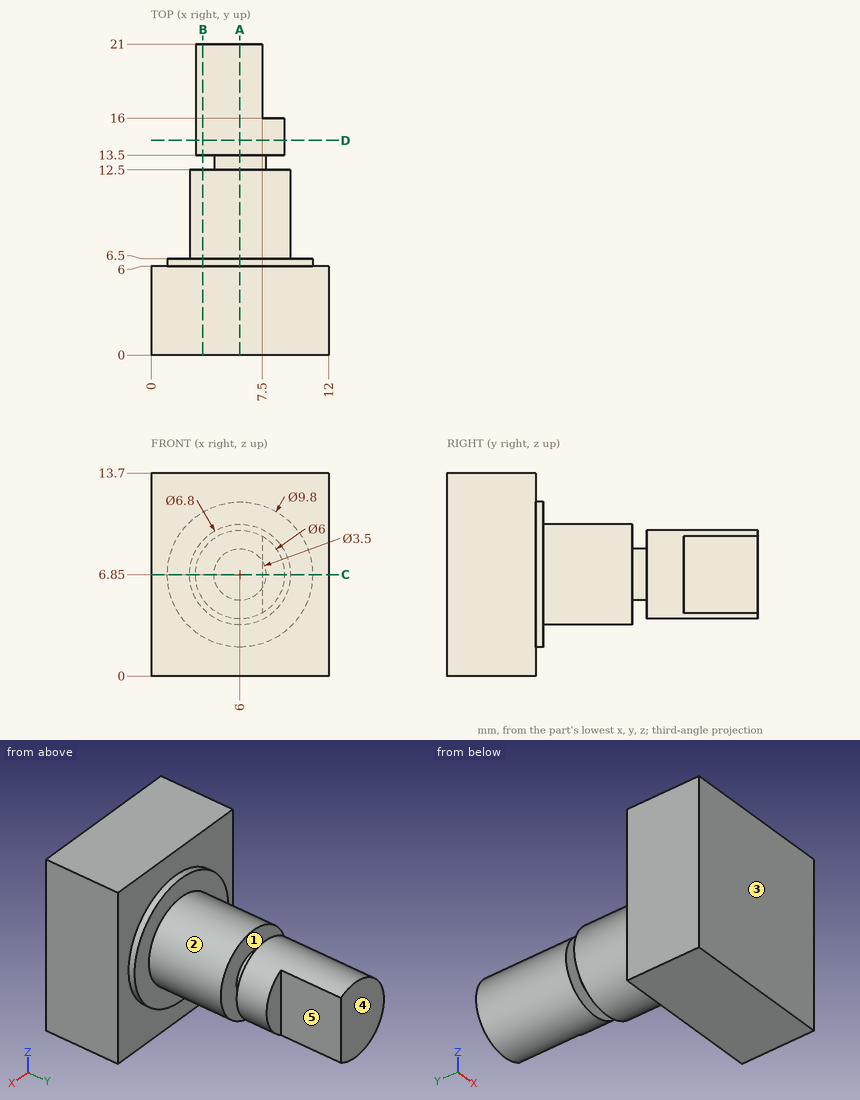
Part print with two shaded views. Sizes in mm from the minimum x, y, z corner. A direction names the side the tool comes from. Give positions to 0.01 mm unless a question says otherwise; leave off trailing zeros. Order: outer loops, then holes, each group sorted by start corner. A loop starts at its lowest first (then second) coordinate and runs counter-clockwise, first axis right, second up.
(1) Tool access for the marked faces 1, 2, 3, 4 and 5: list every direction of +Z, -Z, +X, -X, +Y, -Y with a clear straight run to the whole face (end or side of a thin tool).
(2) Saw through at C-C, the plane z = 6.85. Give the cut face in (x, y), then the cut area to 3 significant figures.
(3) Saw through at D-D, the plane y = 14.5. Give the cut face in (x, z), then the cut area to 3 significant figures.
(4) Drill centre lines: L1, parallel to Y at x = 5.25, z = 1.5; L2, parallel to Y at x = 7.25, z = 4.25; L3, parallel to Y at x = 1.5, z = 5.75. Where is each one in solid material? Low to high.
(5) Saw through at B-B, the plane x = 3.5. Give the cut face in (y, z).
(6) Flat gauge pins, fed straight in: pin 1 (1 mm diameter, centred on y = 10, z = 2, fed in from +X); pin 2 (6 mm diameter, centred on y = 11, z = 1.5, fed in from -X); pin 3 (3 mm diameter, centred on x = 4, y = 13, fed in from -Z); pin 4 (1.5 mm diameter, centred on y = 11.5, z = 6, fed in from +X). Where does each tip first touch, or does it go through?
(7) Saw through at A-A, the plane x = 6. Give the cut face in (y, z).
Results found:
1. face 1: none
1. face 2: +Y
1. face 3: +Z, -Z, +X, -X, -Y
1. face 4: +Z, -Z, +X, -X, +Y
1. face 5: +Z, -Z, +X, +Y
2. outline: (0, 0) - (12, 0) - (12, 6) - (10.9, 6) - (10.9, 6.5) - (9.4, 6.5) - (9.4, 12.5) - (7.75, 12.5) - (7.75, 13.5) - (9, 13.5) - (9, 16) - (7.5, 16) - (7.5, 21) - (3, 21) - (3, 13.5) - (4.25, 13.5) - (4.25, 12.5) - (2.6, 12.5) - (2.6, 6.5) - (1.1, 6.5) - (1.1, 6) - (0, 6) - close
2. area: 159 mm2
3. outline: circle Ø6 at (6, 6.85)
3. area: 28.3 mm2
4. L1: y = 0 to 6
4. L2: y = 0 to 12.5, 13.5 to 21
4. L3: y = 0 to 6.5
5. outline: (0, 0) - (6, 0) - (6, 2.64) - (6.5, 2.64) - (6.5, 4.55) - (12.5, 4.55) - (12.5, 9.15) - (6.5, 9.15) - (6.5, 11.06) - (6, 11.06) - (6, 13.7) - (0, 13.7) - close; (13.5, 5.19) - (21, 5.19) - (21, 8.51) - (13.5, 8.51) - close
6. pin 1: passes through
6. pin 2: stops at x = 3.54
6. pin 3: stops at z = 3.5
6. pin 4: stops at x = 9.4
7. outline: (0, 0) - (6, 0) - (6, 1.95) - (6.5, 1.95) - (6.5, 3.45) - (12.5, 3.45) - (12.5, 5.1) - (13.5, 5.1) - (13.5, 3.85) - (21, 3.85) - (21, 9.85) - (13.5, 9.85) - (13.5, 8.6) - (12.5, 8.6) - (12.5, 10.25) - (6.5, 10.25) - (6.5, 11.75) - (6, 11.75) - (6, 13.7) - (0, 13.7) - close
